from build123d import *

# Parameters (mm, degrees)
PAD_DEPTH            = 3
PAD001_DEPTH         = 10
SKETCH008_W          = 31.5
SKETCH008_H          = 15
PAD004_DEPTH         = 5
SKETCH009_R          = 2.75
POCKET002_DEPTH      = 313.05051685
POCKET002_DEPTH_BACK = 323.05051685
POCKET003_DEPTH      = 353.05051685
POCKET003_DEPTH_BACK = 393.05051685
POCKET004_DEPTH      = 4
PAD005_DEPTH         = 3


with BuildPart() as part:
    # Sketch → Pad (new body)
    with BuildSketch(Plane.XY):
        with BuildLine():
            ThreePointArc((89.9999996665, -10), (100, -1.98e-08), (89.9999997062, 10))
            Line((89.9999997062, 10), (31.5, 10))
            Line((31.5, 10), (31.5, 40))
            Line((31.5, 40), (0, 40))
            Line((0, 40), (0, 10))
            Line((0, 10), (0, -27.3349528301))
            ThreePointArc((5.3000111055, -28.854983356), (2.7568374325, -27.7224688967), (0, -27.3349528301))
            Line((84.6999795851, -78.4799636558), (5.3000111055, -28.854983356))
            ThreePointArc((84.6999795851, -78.4799636557), (98.4799840149, -75.2999878403), (95.2999552657, -61.5199956261))
            Line((42.4359754567, -28.4800082454), (95.2999552657, -61.5199956261))
            ThreePointArc((47.7359245737, -10), (38.1234305175, -17.2431977049), (42.4359754568, -28.4800082453))
            Line((47.7359245737, -10), (89.9999996665, -10))
        make_face()
    pad = extrude(amount=PAD_DEPTH)

    # Sketch001 → Pad001 (join)
    with BuildSketch(Plane.XY):
        with BuildLine():
            ThreePointArc((89.2050015192, -71.2719974118), (91.2719974827, -70.7949983672), (90.7949982537, -68.7280024463))
            Line((90.7949982537, -68.7280024463), (35.2050028881, -33.9842553428))
            ThreePointArc((34.5, -32.7122571332), (34.6880366632, -33.4394105688), (35.2050028881, -33.9842553428))
            Line((34.5, -32.7122571332), (34.5, -1.5))
            Line((34.5, -1.5), (89.9999999914, -1.5))
            ThreePointArc((89.9999999914, -1.5), (91.5, -1.09e-08), (90.0000000131, 1.5))
            Line((90.0000000131, 1.5), (34.5, 1.5))
            Line((34.5, 1.5), (34.5, 40))
            Line((34.5, 40), (31.5, 40))
            Line((31.5, 40), (31.5, -14.334953275))
            ThreePointArc((30.0000000301, -15.8349528301), (31.0606600252, -15.3956131485), (31.5, -14.334953275))
            Line((0, -15.8349528301), (30.0000000301, -15.8349528301))
            Line((0, -18.8349528301), (0, -15.8349528301))
            ThreePointArc((9.8049805408, -21.6469843002), (5.1001265767, -19.5518510506), (0, -18.8349528301))
            Line((89.2050015192, -71.2719974118), (9.8049805408, -21.6469843002))
        make_face()
        with BuildLine():
            Line((15.4013148944, -21.6069503467), (29.2050008044, -30.2342540405))
            ThreePointArc((29.2050008044, -30.2342540405), (30.727152292, -30.2742210781), (31.5, -28.9622573074))
            Line((31.5, -20.3349477146), (31.5, -28.9622573074))
            ThreePointArc((31.5, -20.3349477146), (31.0606583181, -19.2742908047), (29.9999998727, -18.8349528301))
            Line((16.1963133258, -18.8349528301), (29.9999998727, -18.8349528301))
            ThreePointArc((16.1963133258, -18.8349528301), (14.7544400888, -19.9214290586), (15.4013148944, -21.6069503467))
        make_face(mode=Mode.SUBTRACT)
    pad001 = extrude(amount=PAD001_DEPTH)

    # Sketch008 → Pad004 (join)
    with BuildSketch(Plane(origin=(0, 30, 0), x_dir=(1, 0, 0), z_dir=(0, 0, 1))):
        with Locations((15.75, 2.5)):
            Rectangle(SKETCH008_W, SKETCH008_H)
    pad004 = extrude(amount=PAD004_DEPTH)

    # Sketch009 → Pocket002 (cut, two sides)
    with BuildSketch(Plane(origin=(0, 30, 0), x_dir=(1, 0, 0), z_dir=(0, 0, 1))) as pocket002_sk:
        with Locations((21.9, 4)):
            Circle(SKETCH009_R)
    pocket002 = extrude(amount=-POCKET002_DEPTH, mode=Mode.SUBTRACT) + extrude(pocket002_sk.sketch, amount=POCKET002_DEPTH_BACK, mode=Mode.SUBTRACT)

    # Sketch010 → Pocket003 (cut, two sides)
    with BuildSketch(Plane.XZ) as pocket003_sk:
        Polygon((91.5, 3), (30, 10), (91.5, 10), align=None)
    pocket003 = extrude(amount=-POCKET003_DEPTH, mode=Mode.SUBTRACT) + extrude(pocket003_sk.sketch, amount=POCKET003_DEPTH_BACK, mode=Mode.SUBTRACT)

    # Sketch012 → Pocket004 (cut)
    with BuildSketch(Plane(origin=(0, 30, 0), x_dir=(1, 0, 0), z_dir=(0, 0, 1))):
        Polygon((23.9495934556, 7.55), (19.8504065444, 7.55), (17.8008130888, 4), (19.8504065444, 0.45), (23.9495934556, 0.45), (25.9991869112, 4), align=None)
    pocket004 = extrude(amount=POCKET004_DEPTH, mode=Mode.SUBTRACT)

    # Sketch013 → Pad005 (join)
    with BuildSketch(Plane.YZ.offset(31.5)):
        with BuildLine():
            ThreePointArc((40, 20.7833465364), (37.421342396, 25.4323336669), (32.1121450336, 25.706157964))
            Line((32.1121450336, 25.706157964), (0, 10))
            Line((0, 10), (0, 0))
            Line((0, 0), (40, 0))
            Line((40, 20.7833465364), (40, 0))
        make_face()
    pad005 = extrude(amount=PAD005_DEPTH)

    # Mirrored: Pad, Pad001, Pad004, Pocket002, Pocket003, Pocket004, Pad005 across Sketch V_Axis
    add(pad.mirror(Plane(origin=(0, 0, 0), x_dir=(0, 0, 1), z_dir=(1, 0, 0))))
    add(pad001.mirror(Plane(origin=(0, 0, 0), x_dir=(0, 0, 1), z_dir=(1, 0, 0))))
    add(pad004.mirror(Plane(origin=(0, 0, 0), x_dir=(0, 0, 1), z_dir=(1, 0, 0))))
    add(pocket002.mirror(Plane(origin=(0, 0, 0), x_dir=(0, 0, 1), z_dir=(1, 0, 0))), mode=Mode.SUBTRACT)
    add(pocket003.mirror(Plane(origin=(0, 0, 0), x_dir=(0, 0, 1), z_dir=(1, 0, 0))), mode=Mode.SUBTRACT)
    add(pocket004.mirror(Plane(origin=(0, 0, 0), x_dir=(0, 0, 1), z_dir=(1, 0, 0))), mode=Mode.SUBTRACT)
    add(pad005.mirror(Plane(origin=(0, 0, 0), x_dir=(0, 0, 1), z_dir=(1, 0, 0))))


solid = part.part
Verification items for the finished model (mm, model axes). A direction names the side the tool comes from. Coordinates: 2 decimals unless noted, no trailing zeros. Write each loop counter-clockwise with the first axis right and the second up, starting at its lowest first coordinate (ties: lowest second). Pieces come first, ordered by that corner, then holes. Notation, with made-up numbers: (61, 59.25) - (104, 59.25) arc R4 ccw to (104, 66.25) - close; hole circle Ø4 at (-14, 79). An arc over 180 degrees is marked (long way). Answer as a JSON object with one key per item and string values.
(1) Mould release check, pull along Y, two halves, no side actions. Record for faces 5 (the cylindrical face through (-32.98, 37.49, 25.39)), 6 (the flat face through (56, 1.5, 5)), 7 (the flat face through (0, -25, 3)): pulls with the +Y half, pulls with the -Y half, needs draft (parallel to the pull), parting line crosses it, or undercut.
Report:
{"face 5": "parting line crosses it", "face 6": "pulls with the +Y half", "face 7": "undercut"}
(2) Thickness scan on line 1 along X through (y, z) = (34, 4.4); line 2 along Y through (x, z) = (21.9, 4.35); line 3 along X through (y, z) = (3, 7.25). Record the ranges inside material, lowest first.
Report:
{"line 1": "-34.5 to -24.65, -19.15 to 19.15, 24.65 to 34.5", "line 2": "-29.21 to -25.67, -18.83 to -15.83, 25 to 31.25, 36.75 to 40", "line 3": "-34.5 to -31.5, 31.5 to 34.5"}
(3) Gauge pin test, flat ends, axial feed: pin 1 Ø5 at (x, y) = (-52, -42) entering from +Z; pin 2 Ø20.5 at (x, y) = (-11, -28) entering from +Z; pin 3 Ø5 at (x, y) = (-10, 21) entering from +Z; pin 4 Ø8 at (y, z) = (-28, 16.5) entering from -X. Record the tip position at first contact, or that the pin passes through.
Report:
{"pin 1": "z = 7.75", "pin 2": "z = 10", "pin 3": "z = 3", "pin 4": "through"}
(4) Cross-section at D-D on x = -45. Record the cut outline in (y, z).
Report:
{"outline": "(-53.67, 0) - (-30.08, 0) - (-30.08, 3) - (-40.11, 3) - (-40.11, 8.29) - (-43.64, 8.29) - (-43.64, 3) - (-53.67, 3) - close; (-10.38, 0) - (10, 0) - (10, 3) - (1.5, 3) - (1.5, 8.29) - (-1.5, 8.29) - (-1.5, 3) - (-10.38, 3) - close"}
(5) Tool access check on faces 1 (the flat face through (0, 5, 3)), 2 (the flat face through (41.239, -41.293, 5.673)), 3 (the flat face through (56, -1.5, 5)), 4 (the flat face through (-18.81, 32.25, 1.97)). Record the directions out of +Z, -Z, +X, -X, +Y, -Y that give a thin tool (end or side, any length) a straight path to the whole face; none if there is none.
Report:
{"face 1": "+Z", "face 2": "+Z, -Y", "face 3": "+Z, +X", "face 4": "-Z"}
(6) Cross-section at A-A on z = 16.75. Record the cut outline in (x, y), plus the area to 3 significant figures.
Report:
{"outline": "(-34.5, 13.8) - (-31.5, 13.8) - (-31.5, 40) - (-34.5, 40) - close; (31.5, 13.8) - (34.5, 13.8) - (34.5, 40) - (31.5, 40) - close", "area": "157 mm^2"}
(7) Cross-section at C-C on y = -49.5. Record the cut outline in (x, z).
Report:
{"outline": "(-76.07, 0) - (-38.33, 0) - (-38.33, 3) - (-54.37, 3) - (-54.37, 7.23) - (-60.03, 6.58) - (-60.03, 3) - (-76.07, 3) - close; (38.33, 0) - (76.07, 0) - (76.07, 3) - (60.03, 3) - (60.03, 6.58) - (54.37, 7.23) - (54.37, 3) - (38.33, 3) - close"}
(8) Cross-section at B-B on x = 21.9. Record the cut outline in (y, z), plus the area to 3 significant figures.
Report:
{"outline": "(-39.23, 0) - (30.45, 0) - (30.45, 4) - (31.25, 4) - (31.25, 5) - (25, 5) - (25, 3) - (-15.83, 3) - (-15.83, 10) - (-18.83, 10) - (-18.83, 3) - (-25.67, 3) - (-25.67, 10) - (-29.21, 10) - (-29.21, 3) - (-39.23, 3) - close; (36.75, 4) - (37.55, 4) - (37.55, 0) - (40, 0) - (40, 5) - (36.75, 5) - close", "area": "280 mm^2"}
